Autodesk Inventor part; units mm, degrees
ref_plane "YZ Plane" through (0, 0, 0) normal (1, 0, 0) x (0, 1, 0)
ref_plane "XZ Plane" through (0, 0, 0) normal (0, 1, 0) x (-1, 0, 0)
ref_plane "XY Plane" through (0, 0, 0) normal (0, 0, 1) x (1, 0, 0)
sketch "Sketch1" plane through (0, 0, 0) normal (0, 1, 0) x (-1, 0, 0)
  circle A0 centre (0, 0) radius 37.5
  circle A1 centre (0, 0) radius 5
  dimension "d0" = 75
  dimension "d1" = 10
extrude "Extrusion1" add sketch "Sketch1" along normal blind 15
sketch "Sketch2" plane through (0, 15, 0) normal (0, 1, 0) x (1, 0, 0)
  line L0 (-47.5, -47.5) -> (47.5, -47.5)
  line L1 (47.5, -47.5) -> (47.5, 47.5)
  line L2 (47.5, 47.5) -> (-47.5, 47.5)
  line L3 (-47.5, 47.5) -> (-47.5, -47.5)
  line L4 (-47.5, -47.5) -> (47.5, 47.5) construction
  line L5 (47.5, -47.5) -> (-47.5, 47.5) construction
  circle A0 centre (0, 0) radius 37.5
  circle A1 centre (0, 0) radius 5
  line L6 (-10, -5) -> (0, -5)
  line L7 (0, -5) -> (0, 5)
  line L8 (0, 5) -> (-10, 5)
  line L9 (-10, 5) -> (-10, -5)
  line L10 (-10, -5) -> (0, 5) construction
  line L11 (0, -5) -> (-10, 5) construction
  point P0 (-5, 0)
  dimension "d4" = 95
  dimension "d5" = 95
extrude "Extrusion2" add sketch "Sketch2" along normal blind 5 contours L3 L2 L1 L0 | A0 | A1 L6 L9 L8
fillet "Fillet1" radius 5 4 edges at (47.5, 17.5, -47.5) (-47.5, 17.5, -47.5) (47.5, 17.5, 47.5) (-47.5, 17.5, 47.5)
sketch "Sketch4" plane through (0, 0, 0) normal (0, -1, 0) x (1, 0, 0)
  circle A0 centre (0, 0) radius 37.5
  circle A1 centre (0, 0) radius 5
  line L0 (0, 5) -> (-5, 5)
  line L1 (-5, 5) -> (-5, 0)
  line L2 (-5, -5) -> (0, -5)
  line L3 (-5, -5) -> (-5, 0)
sketch "Sketch4 outline for Extrusion3" plane through (0, 0, 0) normal (0, -1, 0) x (1, 0, 0)
  line L0 (-5, 0) -> (-5, -5)
  arc A0 (0, -5) -> (-5, 0) centre (0, 0) cw
  line L1 (-5, -5) -> (0, -5)
  line L2 (-5, 5) -> (-5, 0)
  line L3 (0, 5) -> (-5, 5)
  arc A1 (-5, 0) -> (0, 5) centre (0, 0) cw
extrude "Extrusion3" cut sketch "Sketch4 outline for Extrusion3" against normal blind 10
sketch "Sketch6" plane through (0, 15, 0) normal (0, -1, 0) x (1, 0, 0)
  line L0 (37.5, 38.824232) -> (-37.5, 38.824232)
  line L1 (-37.5, 38.824232) -> (-37.5, -38.824232)
  line L2 (-37.5, -38.824232) -> (37.5, -38.824232)
  line L3 (37.5, -38.824232) -> (37.5, 38.824232)
  line L4 (37.5, 38.824232) -> (-37.5, -38.824232) construction
  line L5 (-37.5, 38.824232) -> (37.5, -38.824232) construction
  point P0 (0, 0)
  dimension "d11" = 75
hole "Hole1" at (37.5, 15, -38.824232) at (-37.5, 15, -38.824232) at (-37.5, 15, 38.824232) at (37.5, 15, 38.824232) direction (0, 1, 0) diameter 5 end through all
properties part number "Saugknopf"
Verification items for the finished model (mm, model axes). A direction names the side the tool comes from. Give positions to 0.01 mm unless a question says otherwise; leave off trailing zeros. Loops run counter-clockwise (first coordinate to the right, second up) from the corner with the lowest first, then second, coordinate; pieces in that order, holes last. Notation, with made-up numbers: M 66.25,-8.75 L 121.25,-8.75 A32 cw 121.25,20.25 Z; hole C 52,37 d8. An arc over 180 degrees is marked long. Return JSON: item names as keys, results as strings.
1) Material ranges on L1, parallel to Z at x = 37.5, y = 17.95; L2, parallel to Y at x = 31, z = 28; L3, parallel to Z at x = 2, y = 12.25, recorded low to high. Write a range as [from, to].
Findings:
{"L1": "z = [-47.5, -41.32], [-36.32, 36.32], [41.32, 47.5]", "L2": "y = [15, 20]", "L3": "z = [-37.45, -4.58], [4.58, 37.45]"}
2) Gauge pin test, flat ends, axial feed: P1, Ø3, axis at x = -29, y = 3.5, coming from the +Z side; P2, Ø4, axis at x = -37.5, z = -38.82, coming from the +Y side; P3, Ø2.5, axis at x = -1.5, y = 4, coming from the +Z side; P4, Ø1.5, axis at x = 4, y = 14, coming from the -Z side. Record the tip position at first contact, or that the pin passes through.
Findings:
{"P1": "stops at z = 25.5", "P2": "passes through", "P3": "stops at z = 37.5", "P4": "stops at z = -37.36"}
3) Mould release check, pull along Z, two halves, no side actions. Record for faces 1 (the flat face through (-1, 20, -11)), 2 (the cylindrical face through (46, 17.54, 46.07)), 3 (the flat face through (-5, 5, 0)), 4 (the flat face through (1, 17, -47.5)): released by +Z, released by -Z, zero draft, split by the parting line, or undercut.
Findings:
{"face 1": "zero draft", "face 2": "released by +Z", "face 3": "undercut", "face 4": "released by -Z"}
4) Tool access check on faces 5 (the flat face through (-1, 17, 47.5)), 6 (the flat face through (-3, 5, -5)). Record the directions out of +Z, -Z, +X, -X, +Y, -Y that give a thin tool (end or side, any length) a straight path to the whole face; none if there is none.
Findings:
{"face 5": "+Z, +X, -X, +Y, -Y", "face 6": "-Y"}
5) Section check A-A, the plane x = -22.5. Enter the section's corners in (y, z), and give its area (4 significant figures).
Findings:
{"outline": "M 0,-30 L 15,-30 L 15,-47.5 L 20,-47.5 L 20,47.5 L 15,47.5 L 15,30 L 0,30 Z", "area": "1,375 mm2"}
6) Section check C-C, the plane z = 31. Enter the section's corners in (x, y).
Findings:
{"outline": "M -47.5,15 L -21.1,15 L -21.1,0 L 21.1,0 L 21.1,15 L 47.5,15 L 47.5,20 L -47.5,20 Z"}
7) Section check B-B, the plane y = 4.5. Enter the section's corners in (x, z).
Findings:
{"outline": "C 0,0 d75; hole M -5,-5 L 0,-5 A5 ccw 0,5 L -5,5 Z"}
